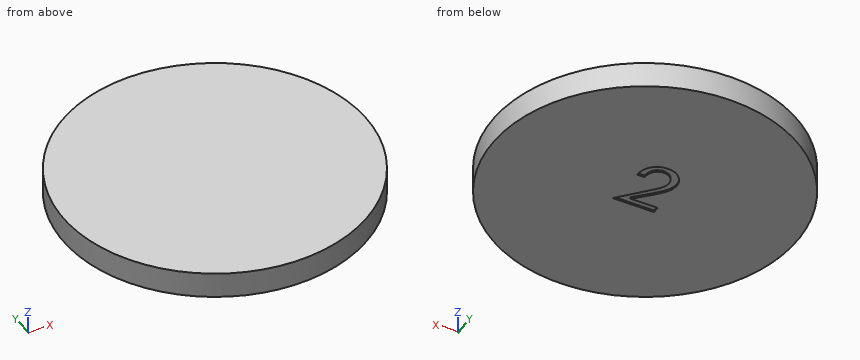
```python
from build123d import *

# Parameters (mm, degrees)
ESQUISSE1_R             = 12.875
BOSS_EXTRU_1_DEPTH      = 2.2
ENL_V_MAT_EXTRU_1_DEPTH = 0.15


with BuildPart() as part:
    # Esquisse1 → Boss.-Extru.1 (new body)
    with BuildSketch(Plane.XY):
        Circle(ESQUISSE1_R)
    extrude(amount=BOSS_EXTRU_1_DEPTH)

    # Esquisse2 → Enlèv. mat.-Extru.1 (cut)
    with BuildSketch(Plane(origin=(0, 0, 0), x_dir=(-1, 0, 0), z_dir=(0, 0, -1))):
        with BuildLine():
            Line((-0.904447115, 1.53394505), (-1.538461538, 1.53394505))
            add(Edge.make_bspline(
                [(-1.538461538, 1.53394505), (-1.535483382, 1.598459427), (-1.529658516, 1.724640697), (-1.50379311, 1.908500904), (-1.461892993, 2.08174412), (-1.409006202, 2.245838985), (-1.338456695, 2.398734226), (-1.257056677, 2.543095198), (-1.158788153, 2.67589638), (-1.047739352, 2.797347851), (-0.927191956, 2.90769124), (-0.797602942, 3.002838248), (-0.661162761, 3.083917548), (-0.517844585, 3.150078794), (-0.36736774, 3.201306183), (-0.210161142, 3.23858307), (-0.045723284, 3.261004233), (0.066369837, 3.263466167), (0.123197115, 3.264714281)],
                knots=[0, 0, 0, 0, 1.154964179, 2.258951466, 3.315045469, 4.34063582, 5.337653555, 6.322213479, 7.300594401, 8.285733883, 9.262436119, 10.219305053, 11.156568068, 12.097250375, 13.037875795, 13.995471444, 14.983774372, 16, 16, 16, 16], degree=3))
            add(Edge.make_bspline(
                [(0.123197115, 3.264714281), (0.182695398, 3.263497204), (0.299447482, 3.261108962), (0.469466636, 3.238635314), (0.630374203, 3.202396573), (0.782217295, 3.15290748), (0.924719266, 3.086826653), (1.058161121, 3.007140463), (1.181260152, 2.911360539), (1.294909804, 2.804188786), (1.395291833, 2.686298975), (1.485957423, 2.565094244), (1.560901311, 2.438116426), (1.623685397, 2.307684161), (1.671998742, 2.17272694), (1.706117474, 2.033793979), (1.726568813, 1.89079087), (1.729360203, 1.794093658), (1.730769231, 1.745283191)],
                knots=[0, 0, 0, 0, 1.156722346, 2.269809107, 3.328396062, 4.361258308, 5.3694338, 6.377253737, 7.377324894, 8.397019439, 9.4098266, 10.385180797, 11.337325354, 12.27255833, 13.196816462, 14.119704983, 15.050871513, 16, 16, 16, 16], degree=3))
            add(Edge.make_bspline(
                [(1.730769231, 1.745283191), (1.728205226, 1.677005358), (1.723112342, 1.541385042), (1.683895559, 1.340742568), (1.617967551, 1.14656255), (1.541814394, 0.988449086), (1.464794664, 0.86064372), (1.394114185, 0.755151869), (1.311082908, 0.641083154), (1.213920187, 0.519201159), (1.106489605, 0.386717178), (0.984523598, 0.247048886), (0.851797199, 0.0973686), (0.757138795, -0.003419183), (0.708133013, -0.055598219)],
                knots=[0, 0, 0, 0, 1.155755081, 2.295677249, 3.447123235, 4.6205014, 5.259503175, 5.973005395, 6.77029923, 7.648035671, 8.612336498, 9.658570495, 10.787814065, 12, 12, 12, 12], degree=3))
            Line((0.708133013, -0.055598219), (-0.521834936, -1.28656777))
            Line((-0.521834936, -1.28656777), (1.794871795, -1.28656777))
            Line((1.794871795, -1.28656777), (1.794871795, -1.863490847))
            Line((1.794871795, -1.863490847), (-1.730769231, -1.863490847))
            Line((-1.730769231, -1.863490847), (0.182291667, 0.24888896))
            add(Edge.make_bspline(
                [(0.182291667, 0.24888896), (0.227858241, 0.297485202), (0.315301331, 0.390742277), (0.438539985, 0.527255661), (0.549728842, 0.653460154), (0.64946069, 0.769264649), (0.735123959, 0.876225683), (0.809023164, 0.97276967), (0.870321749, 1.059352512), (0.933980622, 1.161267724), (0.997060035, 1.283436349), (1.050720551, 1.432464917), (1.082919489, 1.584655413), (1.087467776, 1.687041396), (1.08974359, 1.738271973)],
                knots=[0, 0, 0, 0, 1.341560447, 2.574479018, 3.703506985, 4.728875774, 5.651874962, 6.462761537, 7.177175968, 7.787249671, 8.88179658, 9.938774664, 10.968630673, 12, 12, 12, 12], degree=3))
            add(Edge.make_bspline(
                [(1.08974359, 1.738271973), (1.089182734, 1.770053483), (1.088072967, 1.832939638), (1.072943119, 1.92502887), (1.051630011, 2.014350301), (1.018666087, 2.099467911), (0.978950625, 2.182056297), (0.929273647, 2.261047824), (0.86962043, 2.335709759), (0.803261839, 2.40772195), (0.729867494, 2.472740803), (0.652345526, 2.531053203), (0.569742603, 2.578410458), (0.484317211, 2.619825206), (0.393413852, 2.649185553), (0.299267039, 2.671045841), (0.201137532, 2.686188903), (0.13427309, 2.687249904), (0.100160256, 2.687791204)],
                knots=[0, 0, 0, 0, 0.999432927, 1.977580462, 2.931018689, 3.885672852, 4.844657058, 5.812871023, 6.815890212, 7.849665183, 8.891901864, 9.898878619, 10.897592748, 11.885014695, 12.882178885, 13.896915602, 14.927050508, 16, 16, 16, 16], degree=3))
            add(Edge.make_bspline(
                [(0.100160256, 2.687791204), (0.067729357, 2.68712604), (0.003929265, 2.685817488), (-0.090032164, 2.67231626), (-0.180223502, 2.650333606), (-0.266949004, 2.61984166), (-0.350836809, 2.582223424), (-0.429835719, 2.533489074), (-0.505236946, 2.476796008), (-0.578037313, 2.413166576), (-0.644294043, 2.338516583), (-0.703555767, 2.25373065), (-0.755886208, 2.158716392), (-0.80061588, 2.053640023), (-0.837685545, 1.938225876), (-0.867422698, 1.812614288), (-0.890412391, 1.676750596), (-0.89968233, 1.582427495), (-0.904447115, 1.53394505)],
                knots=[0, 0, 0, 0, 0.911540883, 1.79324023, 2.663162255, 3.518366492, 4.375475705, 5.243419306, 6.122264358, 7.02676621, 7.957780629, 8.921596253, 9.930241338, 11.002848587, 12.128200329, 13.335197372, 14.630280975, 16, 16, 16, 16], degree=3))
        make_face()
    extrude(amount=-ENL_V_MAT_EXTRU_1_DEPTH, mode=Mode.SUBTRACT)


solid = part.part
```
The model under review builds one solid part; all positions refer to its coordinate system, in mm. Round coordinates to 2 decimals unless told otherwise and drop trailing zeros. Loops run counter-clockwise (first coordinate to the right, second up) from the corner with the lowest first, then second, coordinate; pieces in that order, holes last. Notation, with made-up numbers: (47.25, 45) - (72.25, 45) arc R21 ccw to (72.25, 55) - close; hole circle Ø1 at (67, 58.5). An arc over 180 degrees is marked (long way). Use a Markdown table: item, result. Add a question column.
Q1. Add section A-A (z = 0.75). State the section outline as (x, y) points (3 decimals), plus the area to 3 significant figures.
Q2. For probe 1 along X at (y, z) = (-0.25, 1.3); probe 2 along Y at (x, z) = (8, 1); probe 3 along Y at (x, z) = (4.5, 1.1), list the stretches that pass through material, from the lowest coordinate up.
Q3. Add section B-B (x = 4.5). State the section outline as (y, z) points, plus the area to 3 significant figures.
Q4. Add section C-C (y = -8.25). State the section outline as (x, z) points, plus the area to 3 significant figures.
Worked answers:
| question | item | result |
|---|---|---|
| 1 | outline | circle Ø25.75 at (0, 0) |
| 1 | area | 521 mm² |
| 2 | probe 1 | -12.87 to 12.87 |
| 2 | probe 2 | -10.09 to 10.09 |
| 2 | probe 3 | -12.06 to 12.06 |
| 3 | outline | (-12.06, 0) - (12.06, 0) - (12.06, 2.2) - (-12.06, 2.2) - close |
| 3 | area | 53.1 mm² |
| 4 | outline | (-9.88, 0) - (9.88, 0) - (9.88, 2.2) - (-9.88, 2.2) - close |
| 4 | area | 43.5 mm² |
